Work out the finished part from the listing and answer in its coordinate system (mm). Face numbers are marked on the shaded views. A direction names the side the tool comes from. Coordinates: 2 decimals unless noted, no trailing zeros. Order: outer loops, then holes, each group sorted by start corner. A loop starts at its lowest first (then second) coordinate and runs counter-clockwise, first axis right, second up. Notation, with made-up numbers: (-16.5, 56.5) -> (8.5, 56.5) arc R30 ccw to (8.5, 92.5) -> close; hole circle Ø3 at (50, 63.25). An arc over 180 degrees is marked (long way). Use one line per item in the form item = value.
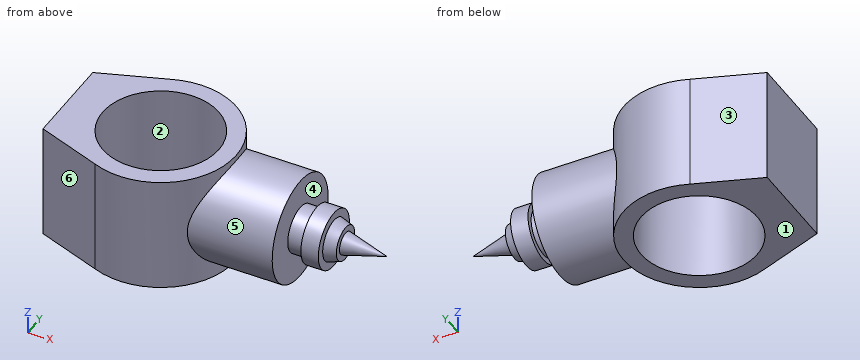
from build123d import *

# Parameters (mm, degrees)
SKETCH1_R           = 50
BOSS_EXTRUDE1_DEPTH = 50
BOSS_EXTRUDE2_REACH = 202
SKETCH2_R           = 45


with BuildPart() as part:
    # Sketch1 → Boss-Extrude1 (new body, symmetric)
    with BuildSketch(Plane.XY):
        with BuildLine():
            Line((-80, -40), (-80, 40))
            Line((-80, 40), (-24.258721248, 60.303519329))
            ThreePointArc((-24.258721248, 60.303519329), (65, 0), (-24.258721248, -60.303519329))
            Line((-24.258721248, -60.303519329), (-80, -40))
        make_face()
        Circle(SKETCH1_R, mode=Mode.SUBTRACT)
    extrude(amount=BOSS_EXTRUDE1_DEPTH, both=True)

    # Sketch2 → Boss-Extrude2 (add, up to next)
    with BuildSketch(Plane(origin=(120, 0, 0), x_dir=(0, 0, -1), z_dir=(1, 0, 0)), mode=Mode.PRIVATE) as boss_extrude2_sk1:
        Circle(SKETCH2_R)
    boss_extrude2_tool1 = extrude(boss_extrude2_sk1.sketch, amount=-BOSS_EXTRUDE2_REACH, mode=Mode.PRIVATE) - part.part
    add(boss_extrude2_tool1.solids().sort_by_distance((120, 0, 0))[0])

    # Sketch3 → Revolve1 (revolve)
    with BuildSketch(Plane.XY):
        Polygon((120, 0), (120, -20), (134, -20), (134, -25), (149, -25), (149, -18), (159, -14.701335797), (159, -9.588406282), (194.736010759, 0), align=None)
    revolve(axis=Axis((0, 0, 0), (1, 0, 0)))


solid = part.part
(1) Section D-D on x = 54 is taken. Write down the section's boundary in (y, z).
Data:
outline = (-36.18, -50) -> (36.18, -50) -> (36.18, -26.76) arc R45 ccw to (36.18, 26.76) -> (36.18, 50) -> (-36.18, 50) -> (-36.18, 26.76) arc R45 ccw to (-36.18, -26.76) -> close
(2) Each of these flat-tipped pins is pushed along its axis until it touches: P1, Ø10, axis at x = 53, z = 9.5, coming from the +Y side; P2, Ø10, axis at x = 101, y = -29, coming from the -Z side; P3, Ø5, axis at x = 11, z = 20.5, coming from the -Y side. Where does it stop, or does it pass through?
Data:
P1 = 44.77
P2 = -38.07
P3 = -64.44
(3) Section A-A on y = 31 is taken. Write down the section's boundary in (x, z).
Data:
outline = (-80, -50) -> (-39.23, -50) -> (-39.23, 50) -> (-80, 50) -> close; (39.23, -50) -> (57.13, -50) -> (57.13, -32.62) -> (120, -32.62) -> (120, 32.62) -> (57.13, 32.62) -> (57.13, 50) -> (39.23, 50) -> close
(4) Which of the six approach directions +Z, -Z, +X, -X, +Y, -Y give full straight-line access (tool end or side, diameter ignored) to the marked faces 4, 5 and 6?
Data:
face_4 = none
face_5 = +X
face_6 = +Z, -Z, -X, -Y
(5) Section C-C on y = -36 is taken. Write down the section's boundary in (x, z).
Data:
outline = (-80, -50) -> (-34.7, -50) -> (-34.7, 50) -> (-80, 50) -> close; (34.7, -50) -> (54.12, -50) -> (54.12, -27) -> (120, -27) -> (120, 27) -> (54.12, 27) -> (54.12, 50) -> (34.7, 50) -> close
(6) The mould has two halves that part along Y. Classify the marked faces 1, 2 and 3: released by +Y, released by -Y, zero draft, split by the parting line, or undercut.
Data:
face_1 = zero draft
face_2 = undercut
face_3 = released by +Y
(7) Section B-B on z = 36 is taken. Write down the section's boundary in (x, y), plus the area to 3 significant figures.
Data:
outline = (-80, -40) -> (-24.26, -60.3) arc R65 ccw to (59.13, -27) -> (120, -27) -> (120, 27) -> (59.13, 27) arc R65 ccw to (-24.26, 60.3) -> (-80, 40) -> close; hole circle Ø100 at (0, 0)
area = 10,500 mm²
(8) Straight lines are drawn through the part: line 1 along Y through (x, z) = (0, -29); line 2 along X through (y, z) = (9, -17); line 3 along Z through (x, y) = (114, -1.5) (3 decimals). For each, find the intervals that lie inside material, in ascending order.
Data:
line_1 = -65 to -50, 50 to 65
line_2 = -80 to -49.18, 49.18 to 149
line_3 = -44.975 to 44.975
